Can you work these out from the model? Positions are in its coordinate system, mm. A direction names the side the tool comes from. Coordinates: 2 decimals unless noted, no trailing zeros. Loops run counter-clockwise (first coordinate to the right, second up) from the corner with the lowest first, then second, coordinate; pieces in that order, holes last. Notation, with made-up numbers: M -2,-10.5 L 41,-10.5 A18 cw 41,12.5 Z; hole C -17.5,33.25 d2. An arc over 180 degrees is marked long. Return JSON: item names as keys, results as strings. Group by question number.
```python
from build123d import *

# Parameters (mm, degrees)
BOSS_EXTRUDE1_DEPTH = 8
SKETCH2_W           = 25
SKETCH2_H           = 5
CUT_EXTRUDE1_DEPTH  = 35
SKETCH3_R           = 2.5
CUT_EXTRUDE2_DEPTH  = 35
FILLET1_R           = 10


with BuildPart() as part:
    # Sketch1 → Boss-Extrude1 (new body)
    with BuildSketch(Plane(origin=(0, 0, 0), x_dir=(1, 0, 0), z_dir=(0, 1, 0))):
        Polygon((0, 0), (0, 8), (70, 8), (70, 18), (100, 18), (100, 0), align=None)
    extrude(amount=BOSS_EXTRUDE1_DEPTH)

    # Sketch2 → Cut-Extrude1 (cut)
    with BuildSketch(Plane.XY):
        with Locations((87.5, 4)):
            Rectangle(SKETCH2_W, SKETCH2_H)
    extrude(amount=-CUT_EXTRUDE1_DEPTH, mode=Mode.SUBTRACT)

    # Sketch3 → Cut-Extrude2 (cut)
    with BuildSketch(Plane(origin=(0, 8, 0), x_dir=(1, 0, 0), z_dir=(0, 1, 0))):
        with Locations(Location((90, 7.5, 0), (0, 0, 270))):
            Circle(SKETCH3_R)
    extrude(amount=-CUT_EXTRUDE2_DEPTH, mode=Mode.SUBTRACT)

    # Fillet1
    fillet1_edges = [part.edges().sort_by_distance(p)[0] for p in [
        (100, 7.25, -18),
        (100, 0.75, -18),
    ]]
    fillet(fillet1_edges, radius=FILLET1_R)


solid = part.part
```
1) Suppose I cut it at A-A, the plane x = 76. List the corners of the cut face in (y, z) for me.
2) If we mould it in two halves opening along X, with no side actions, what happens to faces 4 (the face through (92.48, 7.26, -7.83)), 5 (the face through (62, 8, -7)), 6 (the face through (92.48, 0.76, -7.83)), 7 (the face through (75, 4, -9))? For each: +X half, -X half, draft (parallel to the pull), parting line (faces both ways), or undercut.
3) Suppose I cut it at B-B, the plane z = -7. List the corners of the cut face in (x, y) for me.
4) If I drill on line 1 (X direction, y = 7.25, z = -7.5); line 2 (Z direction, x = 51.5, y = 7); line 3 (X direction, y = 5.5, z = -11.75), over which ranges is the centre line in solid material (lowest first)? Write a range as from..to.
5) Suppose I cut it at C-C, the plane y = 3.75. List the corners of the cut face in (x, z) for me, then the cut area to 3 significant figures.
6) Suppose I cut it at D-D, the plane x = 36. List the corners of the cut face in (y, z) for me.
7) For faces 1 (the face through (70, 4, -13)), 2 (the face through (51, 4, 0)), 3 (the face through (87, 6.5, -9)), which set-ups out of +Z, -Z, +X, -X, +Y, -Y let a thin tool reach every point of the face, with its end or its side?
8) For pin 1 (1 mm diameter, centred on y = 3.5, z = -4.5, fed in from -X); pin 2 (3 mm diameter, centred on x = 90, z = -7.5, fed in from -Y); pin 3 (4 mm diameter, centred on y = 4, z = -10, fed in from +X); pin 4 (2.5 mm diameter, centred on x = 52, y = 4.5, fed in from -Z), each with a flat end and sliding along its axis, tell me the tip position at first contact or that it passes through.
Returned:
{
 "1": {"outline": "M 0,-18 L 1.5,-18 L 1.5,0 L 0,0 Z; M 6.5,-18 L 8,-18 L 8,0 L 6.5,0 Z"},
 "2": {"face 4": "undercut", "face 5": "draft", "face 6": "undercut", "face 7": "+X half"},
 "3": {"outline": "M 0,0 L 87.55,0 L 87.55,1.5 L 75,1.5 L 75,6.5 L 87.55,6.5 L 87.55,8 L 0,8 Z; M 92.45,0 L 100,0 L 100,1.5 L 92.45,1.5 Z; M 92.45,6.5 L 100,6.5 L 100,8 L 92.45,8 Z"},
 "4": {"line 1": "x = 0..87.5, 92.5..100", "line 2": "z = -8..0", "line 3": "x = 70..75"},
 "5": {"outline": "M 0,-8 L 70,-8 L 70,-18 L 75,-18 L 75,0 L 0,0 Z", "area": "650 mm²"},
 "6": {"outline": "M 0,-8 L 8,-8 L 8,0 L 0,0 Z"},
 "7": {"face 1": "-Z, -X, +Y, -Y", "face 2": "+Z, +X, -X, +Y, -Y", "face 3": "+Z, -Z, +X"},
 "8": {"pin 1": "stops at x = 0", "pin 2": "passes through", "pin 3": "stops at x = 75", "pin 4": "stops at z = -8"}
}
